from build123d import *

# Parameters (mm, degrees)
F0_W     = 26
F0_H     = 6
F1_DEPTH = 20
F2_W     = 23
F2_H     = 4
F3_DEPTH = 18
F4_R     = 2
F6_DEPTH = 25
F7_DEPTH = 5


with BuildPart() as f1:
    # F0 (on Top) → F1 (new body)
    with BuildSketch(Plane.XY):
        Rectangle(F0_W, F0_H)
    extrude(amount=F1_DEPTH)

    # F2 (on face) → F3 (cut)
    with BuildSketch(Plane.XY.offset(20)):
        Rectangle(F2_W, F2_H)
    extrude(amount=-F3_DEPTH, mode=Mode.SUBTRACT)

    # F4
    f4_edges = [f1.edges().sort_by_distance(p)[0] for p in [
        (-13, 3, 10),
        (-13, -3, 10),
        (0, -3, 0),
        (13, 0, 0),
        (0, 3, 0),
        (-13, 0, 0),
        (13, -3, 10),
        (13, 3, 10),
    ]]
    fillet(f4_edges, radius=F4_R)

    # F5 (on face) → F6 (cut)
    with BuildSketch(Plane(origin=(0, 0, 0), x_dir=(1, 0, 0), z_dir=(0, 0, -1))):
        with BuildLine():
            Line((-1.7320508076, 1), (1.7320508076, 1))
            ThreePointArc((1.7320508076, 1), (0, 2), (-1.7320508076, 1))
        make_face()
        with BuildLine():
            ThreePointArc((-1.7320508076, -1), (0, -2), (1.7320508076, -1))
            Line((1.7320508076, -1), (-1.7320508076, -1))
        make_face()
        with BuildLine():
            ThreePointArc((1.7320508076, -1), (1.9318516526, -0.5176380902), (2, 0))
            ThreePointArc((2, 0), (1.9318516526, 0.5176380902), (1.7320508076, 1))
            Line((1.7320508076, 1), (-1.7320508076, 1))
            ThreePointArc((-1.7320508076, 1), (-2, 0), (-1.7320508076, -1))
            Line((-1.7320508076, -1), (1.7320508076, -1))
        make_face()
    extrude(amount=-F6_DEPTH, mode=Mode.SUBTRACT)

    # F7 (add): a face of the model
    f7_faces = [f1.faces().sort_by_distance(p)[0] for p in [
        (0, -2.7331667187, 20),
    ]]
    extrude(f7_faces, amount=F7_DEPTH)


solid = f1.part
Check sheet for the modelled part. Datum: model origin and axes. Units: mm. A direction names the side the tool comes from. Round coordinates to 2 decimals unless told otherwise and drop trailing zeros. Order: outer loops, then holes, each group sorted by start corner. A loop starts at its lowest first (then second) coordinate and runs counter-clockwise, first axis right, second up. Notation, with made-up numbers: M 30,67.25 L 57,67.25 A32 cw 57,94.25 Z; hole C -26.75,11.5 d11. An arc over 180 degrees is marked long. One line per item, written item: value. Start each with the question number.
1. Scan lines: line 1 along X through (y, z) = (-0.25, 6.5); line 2 along Y through (x, z) = (1.75, 19.25); line 3 along Z through (x, y) = (11, 0.25). Record each from-to range of solid material in increasing order.
2. Access from +Z, -Z, +X, -X, +Y, -Y to the whole of each face (thin tool, end or side, straight path). Record for faces 1 (the flat face through (-6, 0, 0)), 2 (the flat face through (-7, 0, 2)).
3. Section check C-C on x = -0.5. Enter the section's corners in (y, z).
4. Section check A-A on z = 4. Enter the section's corners in (x, y), and give its area (3 significant figures).
5. Section check B-B on x = 7. Enter the section's corners in (y, z).
6. Gauge pin test, flat ends, axial feed: P1, Ø1.2, axis at x = 6.5, y = -0.5, coming from the +Z side; P2, Ø2, axis at x = 8.5, y = 2.5, coming from the -Z side. Record the tip position at first contact, or that the pin passes through.
Results found:
1. line 1: -13 to -11.5, 11.5 to 13
1. line 2: -3 to -2, 2 to 3
1. line 3: 0 to 2
2. face 1: -Z, +X, -X, +Y, -Y
2. face 2: +Z
3. outline: M -3,2 A2 ccw -1.94,0.23 L -1.94,2 L -2,2 L -2,25 L -3,25 Z; M 1.94,0.23 A2 ccw 3,2 L 3,25 L 2,25 L 2,2 L 1.94,2 Z
4. outline: M -13,-1 A2 ccw -11,-3 L 11,-3 A2 ccw 13,-1 L 13,1 A2 ccw 11,3 L -11,3 A2 ccw -13,1 Z; hole M -11.5,-2 L 11.5,-2 L 11.5,2 L -11.5,2 Z
4. area: 60.6 mm^2
5. outline: M -3,2 A2 ccw -1,0 L 1,0 A2 ccw 3,2 L 3,25 L 2,25 L 2,2 L -2,2 L -2,25 L -3,25 Z
6. P1: z = 2
6. P2: z = 0.06
